Autodesk Inventor part; units mm, degrees
ref_plane "YZ Plane" through (0, 0, 0) normal (1, 0, 0) x (0, 1, 0)
ref_plane "XY Plane" through (0, 0, 0) normal (0, 0, 1) x (1, 0, 0)
sketch "Skizze1" plane through (0, 0, 0) normal (0, 1, 0) x (-1, 0, 0)
  line L0 (0, 0) -> (-78, 0)
  line L1 (-78, 0) -> (-78, -100)
  line L2 (-78, -100) -> (0, -100)
  line L3 (0, -100) -> (0, 0)
  dimension "d0" = 78
  dimension "d1" = 100
extrude "Extrusion1" add sketch "Skizze1" along normal blind 1.5
sketch "Skizze2" plane through (0, 1.5, 0) normal (0, 1, 0) x (1, 0, 0)
  line L0 (78, 100) -> (0, 100)
  line L1 (78, 0) -> (78, 100)
  line L2 (0, 0) -> (78, 0)
  line L3 (0, 100) -> (0, 0)
  point P0 (75, 96)
  point P1 (75, 10)
  point P2 (18, 10)
  point P3 (18, 96)
  dimension "d4" = 4
  dimension "d5" = 3
  dimension "d6" = 10
  dimension "d7" = 3
  dimension "d8" = 18
  dimension "d9" = 10
  dimension "d10" = 4
  dimension "d11" = 18
hole "Bohrung1" at (75, 1.5, -96) at (75, 1.5, -10) at (18, 1.5, -10) at (18, 1.5, -96) direction (0, -1, 0) diameter 3 end through all
sketch "Skizze3" plane through (0, 1.5, 0) normal (0, 1, 0) x (1, 0, 0)
  line L0 (0, 100) -> (0, 0)
  line L1 (0, 15.8637) -> (19.8459, 15.8637)
  line L2 (19.8459, 15.8637) -> (19.8459, 90.2858)
  line L3 (19.8459, 90.2858) -> (0, 90.2858)
  line L4 (0, 90.2858) -> (0, 15.8637)
  dimension "d19" = 15.8637
  dimension "d20" = 74.4222
  dimension "d21" = 19.8459
extrude "Extrusion2" add sketch "Skizze3" along normal blind 18
sketch "Skizze4" plane through (0, 1.5, 0) normal (0, 1, 0) x (1, 0, 0)
  line L0 (78, 0) -> (78, 100)
  line L1 (78, 18) -> (28, 18)
  line L2 (28, 18) -> (28, 88)
  line L3 (28, 88) -> (78, 88)
  line L4 (78, 88) -> (78, 18)
  line L5 (0, 0) -> (78, 0)
  dimension "d24" = 18
  dimension "d25" = 50
  dimension "d26" = 70
extrude "Extrusion3" add sketch "Skizze4" along normal blind 9
sketch "Skizze5" plane through (0, 10.5, 0) normal (0, 1, 0) x (1, 0, 0)
  line L0 (38, 23.0032) -> (78, 23.0032)
  line L1 (78, 23.0032) -> (78, 83.0032)
  line L2 (78, 83.0032) -> (38, 83.0032)
  line L3 (38, 83.0032) -> (38, 23.0032)
  line L4 (78, 18) -> (78, 88)
  line L5 (28, 18) -> (78, 18)
  point P0 (0, 0)
  dimension "d29" = 40
  dimension "d30" = 60
  dimension "d31" = 5.0032
extrude "Extrusion4" add sketch "Skizze5" along normal blind 30
properties part number "jetson"
For this review, take the finished solid that the model builds, in its own axes (mm). A direction names the side the tool comes from. Round coordinates to 2 decimals unless told otherwise and drop trailing zeros. Loops run counter-clockwise (first coordinate to the right, second up) from the corner with the lowest first, then second, coordinate; pieces in that order, holes last.
Q1. Machinability: for faces 4 (the face through (19.846, 10, -53)), 5 (the face through (10, 10, -90.286)), 6 (the face through (58, 25, -83.003)), 7 (the face through (10, 19.5, -54)), 8 (the face through (53, 6, -18)), which of the approach directions +Z, -Z, +X, -X, +Y, -Y give a long, thin tool a straight path to every point of the face, cutting with its end or side? Answer none if there is none.
Result sheet:
face 4: +Z, -Z, +Y
face 5: -Z, +X, -X, +Y
face 6: -Z, +X, +Y
face 7: +Z, -Z, -X, +Y
face 8: +Z, +X, +Y
Q2. To check wall thickness, follow line 1 along X through (y, z) = (0.45, -96); line 2 along Z through (x, y) = (75, 1); line 3 along X through (y, z) = (18, -47). State the ranges of each line that lie inside material, in increasing order.
Result sheet:
line 1: x = 0 to 16.5, 19.5 to 73.5, 76.5 to 78
line 2: z = -100 to -97.5, -94.5 to -11.5, -8.5 to 0
line 3: x = 0 to 19.85, 38 to 78
Q3. Add section A-A on x = 75. Write out the cut boundary in (y, z), plus the area to 3 significant figures.
Result sheet:
outline: (0, -100) - (1.5, -100) - (1.5, -97.5) - (0, -97.5) - close; (0, -94.5) - (1.5, -94.5) - (1.5, -88) - (10.5, -88) - (10.5, -83) - (40.5, -83) - (40.5, -23) - (10.5, -23) - (10.5, -18) - (1.5, -18) - (1.5, -11.5) - (0, -11.5) - close; (0, -8.5) - (1.5, -8.5) - (1.5, 0) - (0, 0) - close
area: 2,570 mm2
Q4. Insertion check: pin 1 Ø6 at (x, z) = (7.5, -40.5) entering from +Y; pin 2 Ø15 at (x, y) = (64.5, 20) entering from +Z; pin 3 Ø10 at (x, y) = (67, 16.5) entering from -Z. Each pin has a flat end and moves straight along its axis. Give the tip position at first contact, or say it passes through.
Result sheet:
pin 1: stops at y = 19.5
pin 2: stops at z = -23
pin 3: stops at z = -83
Q5. Mouldability with a two-part tool opening along Z and no side actions: class faces 1 (the face through (53, 6, -88)), 2 (the face through (16.99, 0.74, -11.11)), 3 (the face through (38, 25, -53)) as +Z half, -Z half, draft (parallel to the pull), parting line (faces both ways), or undercut.
Result sheet:
face 1: -Z half
face 2: undercut
face 3: draft
Q6. Add section C-C on y = 18. Write out the cut boundary in (x, z), plus the area to 3 significant figures.
Result sheet:
outline: (0, -90.29) - (19.85, -90.29) - (19.85, -15.86) - (0, -15.86) - close; (38, -83) - (78, -83) - (78, -23) - (38, -23) - close
area: 3,880 mm2
Q7. Add section D-D on x = 62.5. Write out the cut boundary in (y, z), plus the area to 3 significant figures.
Result sheet:
outline: (0, -100) - (1.5, -100) - (1.5, -88) - (10.5, -88) - (10.5, -83) - (40.5, -83) - (40.5, -23) - (10.5, -23) - (10.5, -18) - (1.5, -18) - (1.5, 0) - (0, 0) - close
area: 2,580 mm2
Q8. Add section B-B on z = -96. Write out the cut boundary in (x, y), plus the area to 3 significant figures.
Result sheet:
outline: (0, 0) - (16.5, 0) - (16.5, 1.5) - (0, 1.5) - close; (19.5, 0) - (73.5, 0) - (73.5, 1.5) - (19.5, 1.5) - close; (76.5, 0) - (78, 0) - (78, 1.5) - (76.5, 1.5) - close
area: 108 mm2
